Verification items for the finished model (mm, model axes). A direction names the side the tool comes from. Coordinates: 2 decimals unless noted, no trailing zeros. Write each loop counter-clockwise with the first axis right and the second up, starting at its lowest first coordinate (ties: lowest second). Pieces come first, ordered by that corner, then holes.
```python
from build123d import *

# Parameters (mm, degrees)
SKETCH1_W           = 240
SKETCH1_H           = 160
BOSS_EXTRUDE1_DEPTH = 4
SKETCH2_W           = 28
SKETCH2_H           = 2
SKETCH2_W_2         = 30
SKETCH2_H_2         = 7.2
BOSS_EXTRUDE3_DEPTH = 35
SKETCH3_R           = 1.65
SKETCH3_R_2         = 4
SKETCH3_R_3         = 11.15
CUT_EXTRUDE1_DEPTH  = 170
SKETCH5_R           = 1.5
CUT_EXTRUDE2_DEPTH  = 4
FILLET1_R           = 25


with BuildPart() as part:
    # Sketch1 → Boss-Extrude1 (new body)
    with BuildSketch(Plane.XY):
        Rectangle(SKETCH1_W, SKETCH1_H)
    extrude(amount=BOSS_EXTRUDE1_DEPTH)

    # Sketch2 → Boss-Extrude3 (add)
    with BuildSketch(Plane(origin=(0, 0, 0), x_dir=(-1, 0, 0), z_dir=(0, 0, -1))):
        with Locations((-70, 79)):
            Rectangle(SKETCH2_W, SKETCH2_H)
        with Locations((-70, -79)):
            Rectangle(SKETCH2_W, SKETCH2_H)
        with Locations((70, -76.4)):
            Rectangle(SKETCH2_W_2, SKETCH2_H_2)
        with Locations((70, 76.4)):
            Rectangle(SKETCH2_W_2, SKETCH2_H_2)
    extrude(amount=BOSS_EXTRUDE3_DEPTH)

    # Sketch3 → Cut-Extrude1 (cut)
    with BuildSketch(Plane.XZ.offset(80)):
        with Locations(Location((78.5, -20, 0), (0, 0, 270))):
            Circle(SKETCH3_R)
        with Locations(Location((61.5, -20, 0), (0, 0, 270))):
            Circle(SKETCH3_R)
        with Locations(Location((70, -20, 0), (0, 0, 270))):
            Circle(SKETCH3_R_2)
        with Locations(Location((-70, -20, 0), (0, 0, 270))):
            Circle(SKETCH3_R_3)
    extrude(amount=-CUT_EXTRUDE1_DEPTH, mode=Mode.SUBTRACT)

    # Sketch5 → Cut-Extrude2 (cut)
    with BuildSketch(Plane.XY.offset(4)):
        with Locations((-110, 70)):
            Circle(SKETCH5_R)
        with Locations((0, 70)):
            Circle(SKETCH5_R)
        with Locations((110, 70)):
            Circle(SKETCH5_R)
        Circle(SKETCH5_R)
        with Locations((110, 0)):
            Circle(SKETCH5_R)
        with Locations((0, -70)):
            Circle(SKETCH5_R)
        with Locations((110, -70)):
            Circle(SKETCH5_R)
        with Locations((-110, 0)):
            Circle(SKETCH5_R)
        with Locations((-110, -70)):
            Circle(SKETCH5_R)
    extrude(amount=-CUT_EXTRUDE2_DEPTH, mode=Mode.SUBTRACT)

    # Fillet1
    fillet1_edges = [part.edges().sort_by_distance(p)[0] for p in [
        (56, -79, 0),
        (84, -79, 0),
        (-85, -76.4, 0),
        (-55, -76.4, 0),
        (-55, 76.4, 0),
        (-85, 76.4, 0),
        (84, 79, 0),
        (56, 79, 0),
    ]]
    fillet(fillet1_edges, radius=FILLET1_R)


solid = part.part
```
1. Sectioned sample at C-C, the plane x = -8. Record the boundary of the cut face in (y, z).
2. Sectioned sample at B-B, the plane z = -5. Record the boundary of the cut face in (x, y), and give its area (3 significant figures).
3. Material ranges on L1, parallel to Y at x = -110, z = 1; L2, parallel to X at y = 70, z = 2.9; L3, parallel to Y at x = -88, z = -10, recorded low to high.
4. Draft check along Z on faces 1 (the flat face through (-67, -72.8, -8)), 2 (the cylindrical face through (-80.885, 76.35, -17.583)), 3 (the cylindrical face through (-92.518, 76.45, -7.129)). Enter one of: pulls with the +Z half, pulls with the -Z half, needs draft (parallel to the pull), parting line crosses it, or undercut.
5. Tool access check on faces 4 (the flat face through (-67, 72.8, -8)), 5 (the flat face through (-70, -76, -35)), 6 (the flat face through (-55, -76, -30)). Record the directions out of +Z, -Z, +X, -X, +Y, -Y that give a thin tool (end or side, any length) a straight path to the whole face; none if there is none.
6. Sectioned sample at D-D, the plane x = 70. Record the boundary of the cut face in (y, z), and give its area (3 significant figures).
7. Sectioned sample at A-A, the plane x = -70. Record the boundary of the cut face in (y, z), and give its area (3 significant figures).
8. Gauge pin test, flat ends, axial feed: P1, Ø3.5, axis at x = -110, y = 70, coming from the -Z side; P2, Ø2.5, axis at x = 0, y = 0, coming from the -Z side; P3, Ø0.6, axis at y = -79, z = -29, coming from the -X side; P4, Ø4.5, axis at x = 61.5, z = -20, coming from the +Y side. Record the tip position at first contact, or that the pin passes through.
Outcome:
1. outline: (-80, 0) - (80, 0) - (80, 4) - (-80, 4) - close
2. outline: (-95, -80) - (-45, -80) - (-45, -72.8) - (-95, -72.8) - close; (-95, 72.8) - (-45, 72.8) - (-45, 80) - (-95, 80) - close; (46, -80) - (94, -80) - (94, -78) - (46, -78) - close; (46, 78) - (94, 78) - (94, 80) - (46, 80) - close
2. area: 912 mm2
3. L1: y = -80 to -71.5, -68.5 to -1.5, 1.5 to 68.5, 71.5 to 80
3. L2: x = -120 to -111.5, -108.5 to -1.5, 1.5 to 108.5, 111.5 to 120
3. L3: y = -80 to -72.8, 72.8 to 80
4. face 1: needs draft
4. face 2: undercut
4. face 3: pulls with the -Z half
5. face 4: -Z, +X, -X
5. face 5: -Z, +X, -X, +Y, -Y
5. face 6: -Z, +Y, -Y
6. outline: (-80, -35) - (-78, -35) - (-78, -24) - (-80, -24) - close; (-80, -16) - (-78, -16) - (-78, 0) - (78, 0) - (78, -16) - (80, -16) - (80, 4) - (-80, 4) - close; (78, -35) - (80, -35) - (80, -24) - (78, -24) - close
6. area: 748 mm2
7. outline: (-80, -35) - (-72.8, -35) - (-72.8, -31.15) - (-80, -31.15) - close; (-80, -8.85) - (-72.8, -8.85) - (-72.8, 0) - (72.8, 0) - (72.8, -8.85) - (80, -8.85) - (80, 4) - (-80, 4) - close; (72.8, -35) - (80, -35) - (80, -31.15) - (72.8, -31.15) - close
7. area: 823 mm2
8. P1: stops at z = 0
8. P2: passes through
8. P3: stops at x = -85
8. P4: stops at y = 80
